For this review, use the dimensioned drawing (mm, ordinates from the lowest corner) and the shaded views. Give positions to 0.01 mm unless a question says otherwise; leave off trailing zeros. Order: outer loops, then holes, each group sorted by start corner. A loop starts at its lowest first (then second) coordinate and runs counter-clockwise, first axis right, second up. Notation, with made-up numbers: M 26,-16 L 33,-16 A20 cw 33,13 Z; hole C 82.5,61.25 d3. An arc over 180 degrees is marked long. Use CSV: the item, a comma, the result in double quotes. Start each with the question number.
(1) Consider section D-D (y = 5). Write out the cut boundary in (x, z).
(2) Consider section A-A (x = 40). Write out the cut boundary in (y, z), and give its area (3 significant figures).
(3) Clearance check with a flat-ended pin moving along its axis: P1, Ø1.5, axis at x = 25, z = 1.5, coming from the -Y side. State where the tip first meets the part, or that it passes through.
(4) Wall thickness on L1, parallel to Y at x = 29.5, z = 2.2; L2, parallel to X at y = 3.5, z = 1.95 (1 decimal); L3, parallel to X at y = 5.5, z = 2.5: over which ranges is each line inside the solid? List them lowest first. Write a range as from..to.
(5) Consider section C-C (z = 2.3). Write out the cut boundary in (x, y).
(6) Consider section B-B (y = 39). Write out the cut boundary in (x, z).
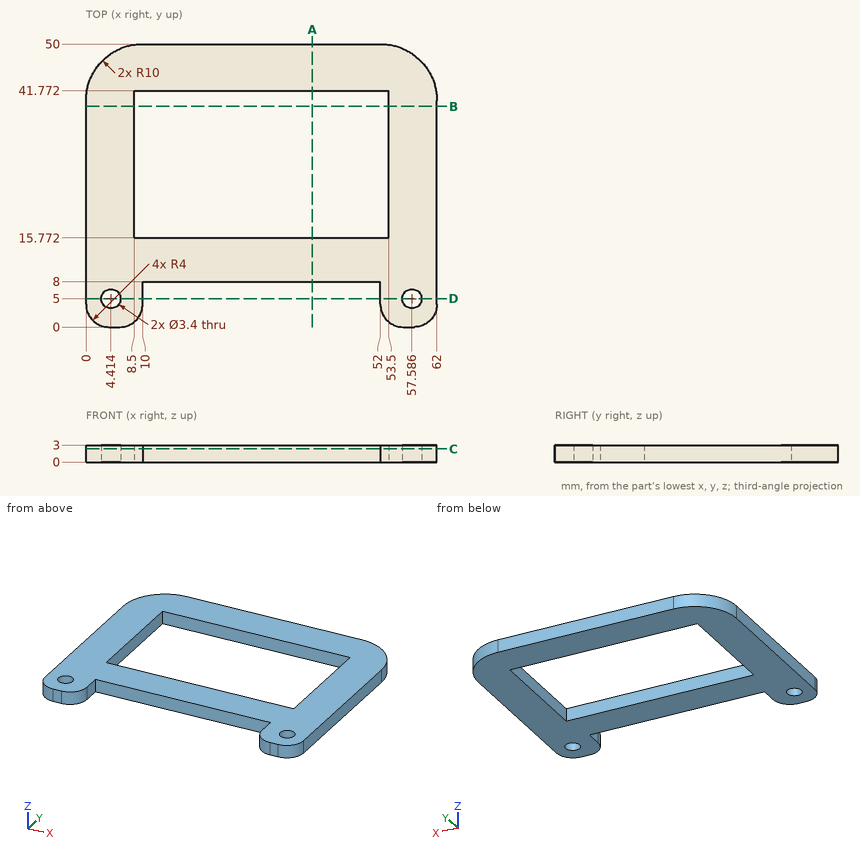
Check result:
1,outline,"M 0,0 L 2.71,0 L 2.71,3 L 0,3 Z; M 6.11,0 L 10,0 L 10,3 L 6.11,3 Z; M 52,0 L 55.89,0 L 55.89,3 L 52,3 Z; M 59.29,0 L 62,0 L 62,3 L 59.29,3 Z"
2,outline,"M 8,0 L 15.77,0 L 15.77,3 L 8,3 Z; M 41.77,0 L 50,0 L 50,3 L 41.77,3 Z"
2,area,"48.0 mm^2"
3,P1,"stops at y = 8"
4,L1,"y = 8..15.77, 41.77..50"
4,L2,"x = 0..3.6, 5.2..10, 52..56.8, 58.4..62"
4,L3,"x = 0..2.79, 6.04..10, 52..55.96, 59.21..62"
5,outline,"M 0,4 A4 ccw 4,0 L 6,0 A4 ccw 10,4 L 10,8 L 52,8 L 52,4 A4 ccw 56,0 L 58,0 A4 ccw 62,4 L 62,40 A10 ccw 52,50 L 10,50 A10 ccw 0,40 Z; hole C 4.41,5 d3.4; hole M 8.5,15.77 L 53.5,15.77 L 53.5,41.77 L 8.5,41.77 Z; hole C 57.59,5 d3.4"
6,outline,"M 0,0 L 8.5,0 L 8.5,3 L 0,3 Z; M 53.5,0 L 62,0 L 62,3 L 53.5,3 Z"
